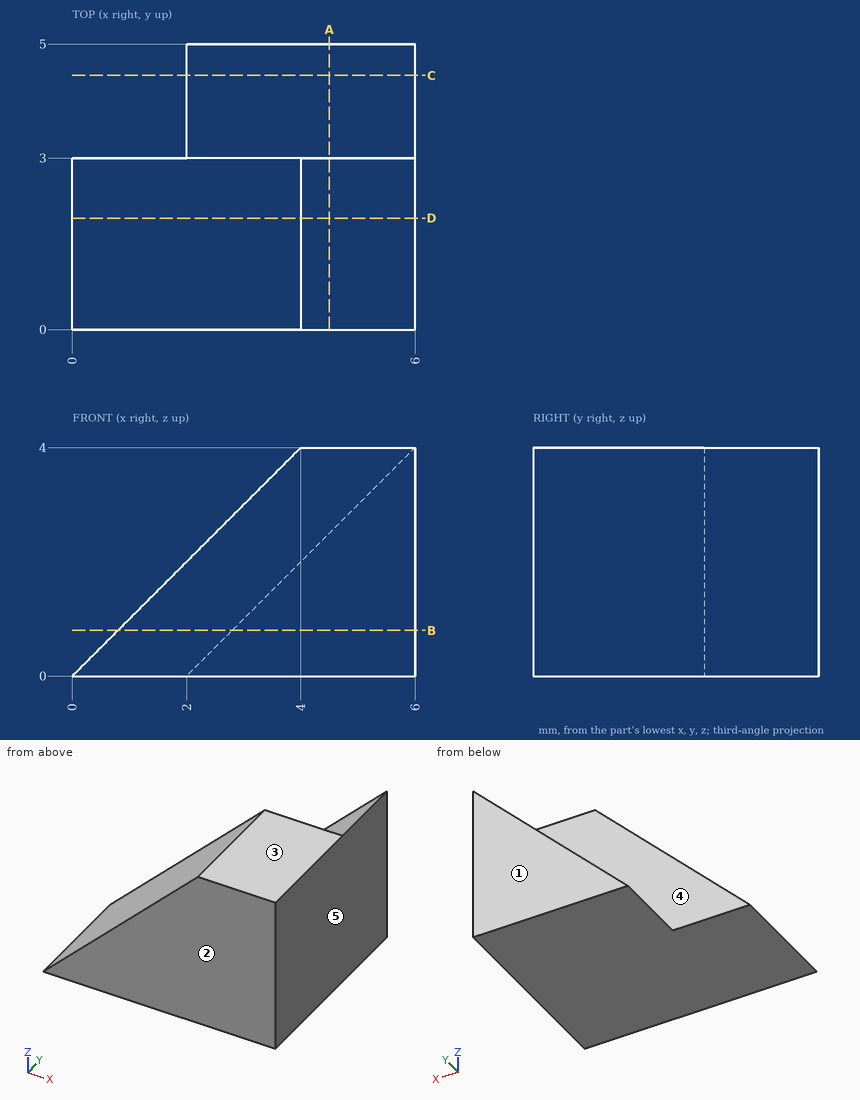
Answer from the drawing. Dimensions are ordinates in mm from the lowest x, y and z of the part. A direction names the side the tool comes from. Give positions to 0.01 mm unless a question says otherwise; leave off trailing zeros. Order: outer loops, then holes, each group sorted by start corner. A loop starts at its lowest first (then second) coordinate and runs counter-clockwise, first axis right, second up. Notation, with made-up numbers: (-18, -16) -> (20, -16) arc R25 cw to (20, 14) -> close; hole circle Ø7 at (56.25, 42). An arc over 180 degrees is marked (long way). One line per item, written item: value.
Item 1: Find section D-D, the plane y = 1.95. Give the vertices of the cut face in (x, z), plus the area to 3 significant figures.
Answer sheet:
outline: (0, 0) -> (6, 0) -> (6, 4) -> (4, 4) -> close
area: 16.0 mm²
Item 2: Flat-ended cylindrical pins translate along their axes: P1, Ø2, axis at x = 2, z = 1.5, coming from the +Y side; P2, Ø3, axis at x = 3.5, y = 1.5, coming from the +Z side. Find the tip coordinate at first contact, or state that the pin passes through.
Answer sheet:
P1: y = 3
P2: z = 4
Item 3: A tool of negligible diameter and unlimited length cuts with its end or side. For the marked faces 4 and 5, from which of +Z, -Z, +X, -X, +Y, -Y can it reach the whole face along a straight path? Write none if from no direction.
Answer sheet:
face 4: +Z, -X, +Y
face 5: +Z, -Z, +X, +Y, -Y
Item 4: Find section A-A, the plane x = 4.5. Give the vertices of the cut face in (y, z), plus the area to 3 significant figures.
Answer sheet:
outline: (0, 0) -> (5, 0) -> (5, 2.5) -> (3, 2.5) -> (3, 4) -> (0, 4) -> close
area: 17.0 mm²
Item 5: Determine the mould class of the marked faces 1, 2 and 3 for opening direction Y: released by +Y, released by -Y, zero draft, split by the parting line, or undercut.
Answer sheet:
face 1: released by +Y
face 2: released by -Y
face 3: zero draft
Item 6: Straight lines are drawn through the part: probe 1 along Y at (x, z) = (1.75, 1.65); probe 2 along Z at (x, y) = (4.25, 4.75); probe 3 along Z at (x, y) = (4.5, 4.4). For each, find the intervals that lie inside material, in ascending order.
Answer sheet:
probe 1: 0 to 3
probe 2: 0 to 2.25
probe 3: 0 to 2.5
Item 7: Find section B-B, the plane z = 0.8. Give the vertices of the cut face in (x, y), plus the area to 3 significant figures.
Answer sheet:
outline: (0.8, 0) -> (6, 0) -> (6, 5) -> (2.8, 5) -> (2.8, 3) -> (0.8, 3) -> close
area: 22.0 mm²
Item 8: Find section C-C, the plane y = 4.45. Give the vertices of the cut face in (x, z), plus the area to 3 significant figures.
Answer sheet:
outline: (2, 0) -> (6, 0) -> (6, 4) -> close
area: 8.00 mm²
